from build123d import *

# Parameters (mm, degrees)
SKETCH1_R               = 3
BOSS_EXTRUDE1_DEPTH     = 18
CUT_EXTRUDE1_START      = -10
CUT_EXTRUDE1_DEPTH      = 10
CUT_EXTRUDE2_DEPTH      = 19.493242009
CUT_EXTRUDE2_DEPTH_BACK = 19.493242009


with BuildPart() as part:
    # Sketch1 → Boss-Extrude1 (new body)
    with BuildSketch(Plane(origin=(0, 0, 0), x_dir=(1, 0, 0), z_dir=(0, 1, 0))):
        with Locations(Location((0, 0, 0), (0, 0, 270))):
            Circle(SKETCH1_R)
    extrude(amount=BOSS_EXTRUDE1_DEPTH)

    # Sketch2 → Cut-Extrude1 (cut)
    with BuildSketch(Plane(origin=(0, 18, 0), x_dir=(1, 0, 0), z_dir=(0, 1, 0)).offset(CUT_EXTRUDE1_START)):
        with BuildLine():
            Line((-2.236067977, -2), (2.236067977, -2))
            ThreePointArc((2.236067977, -2), (0, -3), (-2.236067977, -2))
        make_face()
    extrude(amount=CUT_EXTRUDE1_DEPTH, mode=Mode.SUBTRACT)

    # Sketch3 → Cut-Extrude2 (cut, two sides: drawn at the far end of the back side and taken through both)
    with BuildSketch(Plane(origin=(0, 0, 0), x_dir=(0, 0, -1), z_dir=(1, 0, 0)).offset(-CUT_EXTRUDE2_DEPTH_BACK)):
        Polygon((-2, 8), (-3, 7), (-3, 8), align=None)
    extrude(amount=CUT_EXTRUDE2_DEPTH + CUT_EXTRUDE2_DEPTH_BACK, mode=Mode.SUBTRACT)


solid = part.part
Work out the finished part from the listing and answer in its coordinate system (mm). A direction names the side the tool comes from. Coordinates: 2 decimals unless noted, no trailing zeros. Write each loop counter-clockwise with the first axis right and the second up, starting at its lowest first coordinate (ties: lowest second). Pieces come first, ordered by that corner, then holes. Notation, with made-up numbers: M -10,43 L 0,43 A36 ccw 0,78 Z; hole C -23.75,87 d7. An arc over 180 degrees is marked long. Use one line per item in the form item = value. Start each with the question number.
1. A tool of negligible diameter and unlimited length cuts with its end or side. For faces 1 (the face through (0, 13, 2)), 2 (the face through (0, 0, 0)), from which of +Z, -Z, +X, -X, +Y, -Y can it reach the whole face along a straight path? Write none if from no direction.
2. Each of these flat-tipped pins is pushed along its axis until it touches: P1, Ø1.3, axis at x = 0.5, y = 15, coming from the +Z side; P2, Ø1.5, axis at x = -1, y = 11.5, coming from the -Z side. Where does it stop, or does it pass through?
3. The part is cut by section B-B (y = 1.5). Give the vertices of the cut face in (x, z), plus the area to 3 significant figures.
4. The part is cut by section A-A (x = 0). Give the vertices of the cut face in (y, z).
5. The part is cut by section C-C (z = 1.5). Give the vertices of the cut face in (x, y), plus the area to 3 significant figures.
6. The part is cut by section D-D (y = 11.25). Give the vertices of the cut face in (x, z).
7. Straight lines are drawn through the part: probe 1 along Z at (x, y) = (-1.1, 11.25); probe 2 along Z at (x, y) = (0.4, 13.25); probe 3 along X at (y, z) = (6.25, 0.65). For each, find the intervals that lie inside material, in ascending order. Write a range as from..to.
Evaluation:
q1.face_1 = +Z, +X, -X, +Y
q1.face_2 = +Z, -Z, +X, -X, -Y
q2.P1 = 2
q2.P2 = -2.99
q3.outline = C 0,0 d6
q3.area = 28.3 mm^2
q4.outline = M 0,-3 L 18,-3 L 18,2 L 8,2 L 7,3 L 0,3 Z
q5.outline = M -2.6,0 L 2.6,0 L 2.6,18 L -2.6,18 Z
q5.area = 93.5 mm^2
q6.outline = M -2.24,2 A3 ccw long 2.24,2 Z
q7.probe_1 = -2.79..2
q7.probe_2 = -2.97..2
q7.probe_3 = -2.93..2.93
